```python
from build123d import *

# Parameters (mm, degrees)
PAD002_DEPTH    = 125
PAD003_DEPTH    = 5
SKETCH004_W     = 10.5
SKETCH004_H     = 12.5
POCKET_DEPTH    = 10.4
POCKET001_DEPTH = 15.4
POCKET002_DEPTH = 35
SKETCH016_W     = 18
SKETCH016_H     = 12.5
POCKET008_DEPTH = 5


with BuildPart() as part:
    # Sketch002 → Pad002 (new body)
    with BuildSketch(Plane.XY):
        with BuildLine():
            Line((-9, 15), (9, 15))
            Line((9, 15), (9, 27))
            ThreePointArc((-9, 27), (0, 25.85685), (9, 27))
            Line((-9, 27), (-9, 15))
        make_face()
    extrude(amount=PAD002_DEPTH)

    # Sketch003 → Pad003 (join)
    with BuildSketch(Plane.XY):
        with BuildLine():
            Line((-9, 15), (9, 15))
            Line((9, 15), (9, 55))
            ThreePointArc((9, 55), (0, 64), (-9, 55))
            Line((-9, 55), (-9, 15))
        make_face()
    extrude(amount=-PAD003_DEPTH)

    # Sketch004 → Pocket (cut)
    with BuildSketch(Plane.XZ.offset(-15)):
        with Locations((0, 11.25)):
            Rectangle(SKETCH004_W, SKETCH004_H)
        with Locations((0, 81.25)):
            Rectangle(SKETCH004_W, SKETCH004_H)
    extrude(amount=-POCKET_DEPTH, mode=Mode.SUBTRACT)

    # Sketch008 → Pocket001 (cut)
    with BuildSketch(Plane.XY.offset(25)):
        with BuildLine():
            ThreePointArc((-9, 27), (0, 25.85685), (9, 27))
            Line((9, 27), (9, 23.909518))
            ThreePointArc((-9, 23.909518), (0, 22.85685), (9, 23.909518))
            Line((-9, 27), (-9, 23.909518))
        make_face()
    extrude(amount=POCKET001_DEPTH, mode=Mode.SUBTRACT)

    # Sketch009 → Pocket002 (cut)
    with BuildSketch(Plane.XY.offset(90)):
        with BuildLine():
            ThreePointArc((-9, 27), (0, 25.85685), (9, 27))
            Line((9, 27), (9, 23.909518))
            ThreePointArc((-9, 23.909518), (0, 22.85685), (9, 23.909518))
            Line((-9, 27), (-9, 23.909518))
        make_face()
    extrude(amount=POCKET002_DEPTH, mode=Mode.SUBTRACT)

    # Sketch016 → Pocket008 (cut)
    with BuildSketch(Plane.XZ.offset(-15)):
        with Locations((0, 11.25)):
            Rectangle(SKETCH016_W, SKETCH016_H)
        with Locations((0, 81.25)):
            Rectangle(SKETCH016_W, SKETCH016_H)
    extrude(amount=-POCKET008_DEPTH, mode=Mode.SUBTRACT)


solid = part.part
```
CAD build for the part. Positions are in the model's coordinates, mm. A direction names the side the tool comes from. Round coordinates to 2 decimals unless told otherwise and drop trailing zeros. Loops run counter-clockwise (first coordinate to the right, second up) from the corner with the lowest first, then second, coordinate; pieces in that order, holes last. Notation, with made-up numbers: (72, 16) - (78, 16) arc R30 cw to (78, 47) - close; hole circle Ø3 at (-22, -15). An arc over 180 degrees is marked (long way). Return JSON: item names as keys, results as strings. Group by question number.
Q1. Band-saw the part on A-A on z = 9.5. Give the cut face in (x, y).
Q2. Drill centre lines: line 1 along Z through (x, y) = (5, 19.5); line 2 along Z through (x, y) = (6, 34.5); line 3 along Y through (x, z) = (1, 99). Where is each one in solid material? Low to high. Write a range as [from, to].
Q3. Band-saw the part on C-C on y = 51. Give the cut face in (x, z), plus the area to 3 significant figures.
Q4. Band-saw the part on D-D on z = 37.5. Give the cut face in (x, y).
Q5. Flat gauge pins, fed straight in: pin 1 Ø8 at (x, z) = (3, 19.5) entering from +Y; pin 2 Ø5 at (x, z) = (-1, 11.5) entering from -Y; pin 3 Ø12 at (y, z) = (31, 9) entering from -X; pin 4 Ø3 at (x, z) = (-7, 78.5) entering from -Y. Where does each tip first touch, or does it go through?
Q6. Two-plate mould, pull along X, no slides. Class faces 1 (the face through (0, 64, -2)), 2 (the face through (-7, 20, 11)), 3 (the face through (-5.25, 23, 11)), 4 (the face through (0, 24, 90)): +X half, -X half, draft (parallel to the pull), parting line (faces both ways), or undercut.
Q7. Tool access for faces 5 (the face through (0, 19, 75)), 6 (the face through (0, 15, 107)), 7 (the face through (-0.127, 25.857, 64.853)), 8 (the face through (0, 24, 25)): list every direction of +Z, -Z, +X, -X, +Y, -Y with a clear straight run to the whole face (end or side of a thin tool).
Q8. Band-saw the part on B-B on x = -4. Give the cut face in (y, z).
Solutions:
{
 "1": {"outline": "(-9, 20) - (-5.25, 20) - (-5.25, 25.4) - (5.25, 25.4) - (5.25, 20) - (9, 20) - (9, 27) arc R36 cw to (-9, 27) - close"},
 "2": {"line 1": "z = [-5, 5], [17.5, 75], [87.5, 125]", "line 2": "z = [-5, 0]", "line 3": "y = [15, 22.87]"},
 "3": {"outline": "(-9, -5) - (9, -5) - (9, 0) - (-9, 0) - close", "area": "90.0 mm^2"},
 "4": {"outline": "(-9, 15) - (9, 15) - (9, 23.91) arc R39 cw to (-9, 23.91) - close"},
 "5": {"pin 1": "stops at y = 26.54", "pin 2": "stops at y = 25.4", "pin 3": "stops at x = -9", "pin 4": "stops at y = 20"},
 "6": {"face 1": "parting line", "face 2": "draft", "face 3": "undercut", "face 4": "undercut"},
 "7": {"face 5": "-Y", "face 6": "+Z, -Z, +X, -X, -Y", "face 7": "+Z, +Y", "face 8": "+Y"},
 "8": {"outline": "(15, -5) - (63.06, -5) - (63.06, 0) - (26.08, 0) - (26.08, 25) - (23.06, 25) - (23.06, 40.4) - (26.08, 40.4) - (26.08, 90) - (23.06, 90) - (23.06, 125) - (15, 125) - (15, 87.5) - (25.4, 87.5) - (25.4, 75) - (15, 75) - (15, 17.5) - (25.4, 17.5) - (25.4, 5) - (15, 5) - close"}
}
